from build123d import *

# Parameters (mm, degrees)
SKETCH_1_W          = 100
SKETCH_1_H          = 26
EXTRUDE_1_DEPTH     = 13.5
SKETCH_2_W          = 19.106704299
SKETCH_2_H          = 9.5
CUT_EXTRUDE_1_DEPTH = 105.202927022
CHAMFER_1_SIZE      = 2.2
CHAMFER_2_SIZE      = 4
SKETCH_3_R          = 1.5
CUT_EXTRUDE_2_DEPTH = 105.202927022
SKETCH_4_W          = 13.5
SKETCH_4_H          = 12
CUT_EXTRUDE_3_DEPTH = 82.450905458
CHAMFER_3_SIZE      = 2


with BuildPart() as part:
    # Эскиз1 → Вытянуть1 (new body)
    with BuildSketch(Plane(origin=(0, 0, 0), x_dir=(1, 0, 0), z_dir=(0, 1, 0))):
        with Locations((26, -13)):
            Rectangle(SKETCH_1_W, SKETCH_1_H)
    extrude(amount=EXTRUDE_1_DEPTH)

    # Эскиз2 → Вырез-Вытянуть1 (cut, through all)
    with BuildSketch(Plane(origin=(76, 0, 0), x_dir=(0, 0, -1), z_dir=(1, 0, 0))):
        with Locations((-18.569613205, 8.75)):
            Rectangle(SKETCH_2_W, SKETCH_2_H)
    extrude(amount=-CUT_EXTRUDE_1_DEPTH, mode=Mode.SUBTRACT)

    # Фаска1
    chamfer_1_edges = [part.edges().sort_by_distance(p)[0] for p in [
        (26, 13.5, 0),
        (26, 13.5, 9.016261055),
    ]]
    chamfer(chamfer_1_edges, length=CHAMFER_1_SIZE)

    # Фаска2
    chamfer_2_edges = [part.edges().sort_by_distance(p)[0] for p in [
        (26, 0, 0),
    ]]
    chamfer(chamfer_2_edges, length=CHAMFER_2_SIZE)

    # Эскиз3 → Вырез-Вытянуть2 (cut, through all)
    with BuildSketch(Plane(origin=(76, 0, 0), x_dir=(0, 0, -1), z_dir=(1, 0, 0))):
        with Locations((-4.508130527, 9.5)):
            Circle(SKETCH_3_R)
    extrude(amount=-CUT_EXTRUDE_2_DEPTH, mode=Mode.SUBTRACT)

    # Эскиз4 → Вырез-Вытянуть3 (cut, through all)
    with BuildSketch(Plane(origin=(0, 13.5, 0), x_dir=(1, 0, 0), z_dir=(0, 1, 0))):
        with Locations((-12.25, -6)):
            Rectangle(SKETCH_4_W, SKETCH_4_H)
        with Locations((64.25, -6)):
            Rectangle(SKETCH_4_W, SKETCH_4_H)
        with Locations((13.25, -6)):
            Rectangle(SKETCH_4_W, SKETCH_4_H)
        with Locations((38.75, -6)):
            Rectangle(SKETCH_4_W, SKETCH_4_H)
    extrude(amount=-CUT_EXTRUDE_3_DEPTH, mode=Mode.SUBTRACT)

    # Фаска3
    chamfer_3_edges = [part.edges().sort_by_distance(p)[0] for p in [
        (26, 0, 26),
    ]]
    chamfer(chamfer_3_edges, length=CHAMFER_3_SIZE)


solid = part.part
The listing builds one solid part. Answer for the finished solid, in the listing's coordinates (mm). A direction names the side the tool comes from. Coordinates: 2 decimals unless noted, no trailing zeros. Loops run counter-clockwise (first coordinate to the right, second up) from the corner with the lowest first, then second, coordinate; pieces in that order, holes last. Notation, with made-up numbers: (-25.5, -7) -> (-8.5, -7) arc R21 cw to (-8.5, 30) -> close; hole circle Ø3 at (-19.5, 54.25). An arc over 180 degrees is marked (long way). Answer in a Markdown table with one row per item. Add a question column.
1. The part is cut by section B-B, the plane y = 9.5. Count the separate pieces of the cut face and the enclosed holes in it, then the cut area to 3 significant figures.
2. The part is cut by section A-A, the plane x = 51.5. Write down the section's boundary in (y, z), then the cut area to 3 significant figures.
3. The part is cut by section D-D, the plane z = 18.5. Write down the section's boundary in (x, y), then the cut area to 3 significant figures.
4. Consider line 1 (X direction, y = 13.25, z = 4.5); line 2 (Y direction, x = 72.5, z = 19); line 3 (Z direction, x = -17, y = 3.75). Determine where each line is inside the solid, lowest interval first. Write a range as [from, to].
5. Determine the mould class of faces 4 (the flat face through (45.5, 7, 6)), 5 (the flat face through (-21.5, 12.4, 1.1)), 6 (the flat face through (32, 7, 6)) for opening direction X: +X half, -X half, draft (parallel to the pull), parting line (faces both ways), or undercut.
6. The part is cut by section C-C, the plane x = 63.5. Write down the section's boundary in (y, z), then the cut area to 3 significant figures.
7. Flat-ended cylindrical pins translate along their axes: P1, Ø8, axis at y = 11, z = 13.5, coming from the -X side; P2, Ø4.5, axis at x = 67, y = 2.5, coming from the -Z side; P3, Ø4, axis at x = 73.5, y = 6.5, coming from the +Z side; P4, Ø2, axis at x = 26.5, z = 18, coming from the +Y side. Find the tip coordinate at first contact, or state that the pin passes through.
8. For faces 1 (the flat face through (1, 8, 9.016)), 2 (the flat face through (73.5, 12.4, 1.1)), 3 (the flat face through (-19, 7, 6)), determine the directions among +Z, -Z, +X, -X, +Y, -Y from which every point of the face is accessible in a straight line to the end or side of a thin tool.
Answer below:
| question | item | result |
|---|---|---|
| 1 | separate pieces | 10 |
| 1 | enclosed holes | 0 |
| 1 | area | 277 mm2 |
| 2 | outline | (0, 4) -> (4, 0) -> (11.3, 0) -> (13.5, 2.2) -> (13.5, 6.82) -> (11.3, 9.02) -> (4, 9.02) -> (4, 26) -> (2, 26) -> (0, 24) -> close; hole circle Ø3 at (9.5, 4.51) |
| 2 | area | 168 mm2 |
| 3 | outline | (-24, 0) -> (76, 0) -> (76, 4) -> (-24, 4) -> close |
| 3 | area | 400 mm2 |
| 4 | line 1 | [-24, -19], [-5.5, 6.5], [20, 32], [45.5, 57.5], [71, 76] |
| 4 | line 2 | [0, 4] |
| 4 | line 3 | [12, 26] |
| 5 | face 4 | undercut |
| 5 | face 5 | draft |
| 5 | face 6 | undercut |
| 6 | outline | (0, 12) -> (4, 12) -> (4, 26) -> (2, 26) -> (0, 24) -> close |
| 6 | area | 54.0 mm2 |
| 7 | P1 | through |
| 7 | P2 | z = 12 |
| 7 | P3 | z = 9.02 |
| 7 | P4 | y = 4 |
| 8 | face 1 | +Z, +X, -X, +Y |
| 8 | face 2 | -Z, +X, -X, +Y |
| 8 | face 3 | -Z, +Y, -Y |
